CAD build for the part. Positions are in the model's coordinates, mm. Face numbers are marked on the shaded views. A direction names the side the tool comes from. Give positions to 0.01 mm unless a question says otherwise; leave off trailing zeros. Write each loop counter-clockwise with the first axis right and the second up, starting at its lowest first coordinate (ties: lowest second). Pieces come first, ordered by that corner, then holes. Notation, with made-up numbers: (-25, 44) - (20, 44) arc R35 cw to (20, 82) - close; hole circle Ø9 at (87, 49.5). An arc over 180 degrees is marked (long way). Answer as a JSON object with one key per item and string values.
from build123d import *

# Parameters (mm, degrees)
BOSS_EXTRUDE1_DEPTH = 1.5
BOSS_EXTRUDE2_DEPTH = 3.5
SKETCH3_R           = 1.15
CUT_EXTRUDE1_DEPTH  = 12.090536506


with BuildPart() as part:
    # Sketch1 → Boss-Extrude1 (new body)
    with BuildSketch(Plane(origin=(0, 0, 0), x_dir=(1, 0, 0), z_dir=(0, 1, 0))):
        with BuildLine():
            Line((0, 7), (5, 7))
            ThreePointArc((5, 7), (6.414213562, 6.414213562), (7, 5))
            Line((7, 5), (7, 0))
            Line((7, 0), (7, -5))
            ThreePointArc((7, -5), (6.414213562, -6.414213562), (5, -7))
            Line((5, -7), (0, -7))
            Line((0, -7), (-5, -7))
            ThreePointArc((-5, -7), (-6.414213562, -6.414213562), (-7, -5))
            Line((-7, -5), (-7, 0))
            Line((-7, 0), (-7, 5))
            ThreePointArc((-7, 5), (-6.414213562, 6.414213562), (-5, 7))
            Line((-5, 7), (0, 7))
        make_face()
    extrude(amount=BOSS_EXTRUDE1_DEPTH)

    # Sketch2 → Boss-Extrude2 (add)
    with BuildSketch(Plane(origin=(0, 1.5, 0), x_dir=(1, 0, 0), z_dir=(0, 1, 0))):
        with BuildLine():
            Line((0, 7), (5, 7))
            ThreePointArc((5, 7), (6.414213562, 6.414213562), (7, 5))
            Line((7, 5), (7, 0))
            Line((7, 0), (7, -5))
            ThreePointArc((7, -5), (6.414213562, -6.414213562), (5, -7))
            Line((5, -7), (0, -7))
            Line((0, -7), (-5, -7))
            ThreePointArc((-5, -7), (-6.414213562, -6.414213562), (-7, -5))
            Line((-7, -5), (-7, 0))
            Line((-7, 0), (-7, 5))
            ThreePointArc((-7, 5), (-6.414213562, 6.414213562), (-5, 7))
            Line((-5, 7), (0, 7))
        make_face()
        with BuildLine():
            Line((0, 5), (3.15, 5))
            ThreePointArc((3.15, 5), (3.691852455, 3.691852455), (5, 3.15))
            Line((5, 3.15), (5, 0))
            Line((5, 0), (5, -3.15))
            ThreePointArc((5, -3.15), (3.691852455, -3.691852455), (3.15, -5))
            Line((3.15, -5), (0, -5))
            Line((0, -5), (-3.15, -5))
            ThreePointArc((-3.15, -5), (-3.691852455, -3.691852455), (-5, -3.15))
            Line((-5, -3.15), (-5, 0))
            Line((-5, 0), (-5, 3.15))
            ThreePointArc((-5, 3.15), (-3.691852455, 3.691852455), (-3.15, 5))
            Line((-3.15, 5), (0, 5))
        make_face(mode=Mode.SUBTRACT)
    extrude(amount=BOSS_EXTRUDE2_DEPTH)

    # Sketch3 → Cut-Extrude1 (cut, through all)
    with BuildSketch(Plane(origin=(0, 5, 0), x_dir=(1, 0, 0), z_dir=(0, 1, 0))):
        with Locations(Location((5, 5, 0), (0, 0, 270))):
            Circle(SKETCH3_R)
        with Locations(Location((5, -5, 0), (0, 0, 270))):
            Circle(SKETCH3_R)
        with Locations(Location((-5, -5, 0), (0, 0, 270))):
            Circle(SKETCH3_R)
        with Locations(Location((-5, 5, 0), (0, 0, 270))):
            Circle(SKETCH3_R)
    extrude(amount=-CUT_EXTRUDE1_DEPTH, mode=Mode.SUBTRACT)


solid = part.part
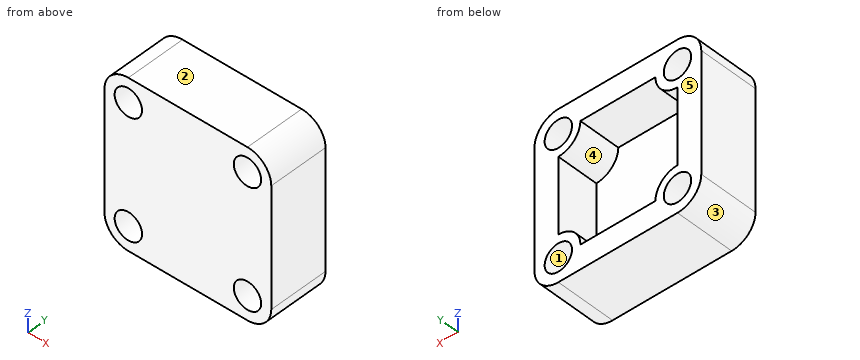
Item 1: Which spindle directions (+Z, -Z, +X, -X, +Y, -Y) get a long thin tool onto all of the face, cutting with end or side? Do the marked faces 4 and 5. Say none if no direction does.
Entries:
{"face 4": "+Y", "face 5": "+Z, -Z, +X, -X, +Y"}
Item 2: Mould opens along Z. For the marked faces 1, 2 and 3 say: +Z half, -Z half, draft (parallel to the pull), parting line (faces both ways), or undercut.
Entries:
{"face 1": "undercut", "face 2": "+Z half", "face 3": "-Z half"}
Item 3: Cut at C-C (y = 0.9). Give the cut face in (x, z).
Entries:
{"outline": "(-7, -5) arc R2 ccw to (-5, -7) - (5, -7) arc R2 ccw to (7, -5) - (7, 5) arc R2 ccw to (5, 7) - (-5, 7) arc R2 ccw to (-7, 5) - close; hole circle Ø2.3 at (-5, -5); hole circle Ø2.3 at (-5, 5); hole circle Ø2.3 at (5, -5); hole circle Ø2.3 at (5, 5)"}
Item 4: Cut at D-D (x = -5.5). Give the cut face in (y, z), and give its area (3 significant figures).
Entries:
{"outline": "(0, -6.94) - (5, -6.94) - (5, -6.04) - (0, -6.04) - close; (0, -3.96) - (5, -3.96) - (5, 3.96) - (0, 3.96) - close; (0, 6.04) - (5, 6.04) - (5, 6.94) - (0, 6.94) - close", "area": "48.7 mm2"}
Item 5: Probe line 1 (X direction, y = 4.5, z = -3); line 2 (X direction, y = 2.3, z = 4.75). List the from-to ranges inside material, lowest first. Write a range as from..to.
Entries:
{"line 1": "-7..-5, 5..7", "line 2": "-7..-6.12, -3.88..-3.17, 3.17..3.88, 6.12..7"}
Item 6: Cut at B-B (x = 2). Give the cut face in (y, z), and give its area (3 significant figures).
Entries:
{"outline": "(0, -7) - (5, -7) - (5, -5) - (1.5, -5) - (1.5, 5) - (5, 5) - (5, 7) - (0, 7) - close", "area": "35.0 mm2"}
Item 7: Cut at A-A (y = 4.05). Give the cut face in (x, z), and give its area (3 significant figures).
Entries:
{"outline": "(-7, -5) arc R2 ccw to (-5, -7) - (5, -7) arc R2 ccw to (7, -5) - (7, 5) arc R2 ccw to (5, 7) - (-5, 7) arc R2 ccw to (-7, 5) - close; hole circle Ø2.3 at (-5, -5); hole circle Ø2.3 at (-5, 5); hole (-5, -3.15) arc R1.85 cw to (-3.15, -5) - (3.15, -5) arc R1.85 cw to (5, -3.15) - (5, 3.15) arc R1.85 cw to (3.15, 5) - (-3.15, 5) arc R1.85 cw to (-5, 3.15) - close; hole circle Ø2.3 at (5, -5); hole circle Ø2.3 at (5, 5)", "area": "86.7 mm2"}
Item 8: Flat gauge pins, fed straight in: P1, Ø2, axis at x = 5, z = 5, coming from the -Y side; P2, Ø3, axis at x = -0.5, z = 0, coming from the +Y side. Where does each tip first touch, or does it go through?
Entries:
{"P1": "through", "P2": "y = 1.5"}
